The listing builds one solid part. Answer for the finished solid, in the listing's coordinates (mm). A direction names the side the tool comes from. Coordinates: 2 decimals unless noted, no trailing zeros. Loops run counter-clockwise (first coordinate to the right, second up) from the corner with the lowest first, then second, coordinate; pieces in that order, holes last. Notation, with made-up numbers: (-28.75, -10.5) - (-24.75, -10.5) arc R28 ccw to (-24.75, 12.5) - close; hole circle Ø5 at (69, 56). An arc over 180 degrees is marked (long way). One line per question, with ' | ' between items.
from build123d import *

# Parameters (mm, degrees)
SKETCH_1_R            = 2.75
EXTRUDE_248_DEPTH     = 3
CUT_EXTRUDE_378_DEPTH = 1.3
SKETCH_3_R            = 1.5
EXTRUDE_479_DEPTH     = 16


with BuildPart() as part:
    # 草图1 → Extrude 248 (new body)
    with BuildSketch(Plane(origin=(0, 0, 0), x_dir=(1, 0, 0), z_dir=(0, 1, 0))):
        Circle(SKETCH_1_R)
    extrude(amount=EXTRUDE_248_DEPTH)

    # 草图2 → Cut-Extrude 378 (cut)
    with BuildSketch(Plane(origin=(0, 3, 0), x_dir=(1, 0, 0), z_dir=(0, 1, 0))):
        Polygon((1.443375673, 0), (0.721687836, 1.25), (-0.721687836, 1.25), (-1.443375673, 0), (-0.721687836, -1.25), (0.721687836, -1.25), align=None)
    extrude(amount=-CUT_EXTRUDE_378_DEPTH, mode=Mode.SUBTRACT)

    # 草图3 → Extrude 479 (add)
    with BuildSketch(Plane.XZ):
        Circle(SKETCH_3_R)
    extrude(amount=EXTRUDE_479_DEPTH)


solid = part.part
Item 1: Find section A-A, the plane x = 0. Write down the section's boundary in (y, z), plus the area to 4 significant figures.
Taken from the geometry:
outline: (-16, -1.5) - (0, -1.5) - (0, -2.75) - (3, -2.75) - (3, -1.25) - (1.7, -1.25) - (1.7, 1.25) - (3, 1.25) - (3, 2.75) - (0, 2.75) - (0, 1.5) - (-16, 1.5) - close | area: 61.25 mm2
Item 2: Which of the six approach directions +Z, -Z, +X, -X, +Y, -Y give full straight-line access (tool end or side, diameter ignored) to faces 1 (the face through (0, -16, 0)), 2 (the face through (1.088, 2.359, -0.616)), 3 (the face through (-1.5, -7.89, 0.07))?
Taken from the geometry:
face 1: +Z, -Z, +X, -X, -Y | face 2: +Y | face 3: -Y
Item 3: The mould has two halves that part along X. Classify faces 4 (the face through (0, 1.7, 0)), 5 (the face through (1.2, 0, 1.2)), 6 (the face through (-0.596, 1.479, 2.685)): pulls with the +X half, pulls with the -X half, needs draft (parallel to the pull), parting line crosses it, or undercut.
Taken from the geometry:
face 4: undercut | face 5: needs draft | face 6: parting line crosses it
Item 4: Find section B-B, the plane z = 0.4. Write down the section's boundary in (x, y), plus the area to 3 significant figures.
Taken from the geometry:
outline: (-2.72, 0) - (-1.45, 0) - (-1.45, -16) - (1.45, -16) - (1.45, 0) - (2.72, 0) - (2.72, 3) - (1.21, 3) - (1.21, 1.7) - (-1.21, 1.7) - (-1.21, 3) - (-2.72, 3) - close | area: 59.4 mm2
Item 5: Find section C-C, the plane y = -3.5. Write down the section's boundary in (x, z), plus the area to 3 significant figures.
Taken from the geometry:
outline: circle Ø3 at (0, 0) | area: 7.07 mm2
Item 6: Find section D-D, the plane x = -1.8. Write down the section's boundary in (y, z).
Taken from the geometry:
outline: (0, -2.08) - (3, -2.08) - (3, 2.08) - (0, 2.08) - close
Item 7: Find the intervals of material crossed by line 1 (Y direction, x = -1, z = -0.6); line 2 (Y direction, x = -2.35, z = -0.1); line 3 (X direction, y = 2.25, z = 0.8), in increasing order. Write a range as [from, to].
Taken from the geometry:
line 1: y = [-16, 1.7] | line 2: y = [0, 3] | line 3: x = [-2.63, -0.98], [0.98, 2.63]
Item 8: Each of these flat-tipped pins is pushed along its axis until it touches: pin 1 Ø3 at (x, y) = (-1.5, -12.5) entering from -Z; pin 2 Ø1.5 at (y, z) = (-12, 2) entering from +X; pin 3 Ø3 at (x, y) = (0.5, -4.5) entering from +Z. Where does it stop, or does it pass through?
Taken from the geometry:
pin 1: stops at z = -1.5 | pin 2: stops at x = 0.83 | pin 3: stops at z = 1.5
